Design review of the part shown in the three views and the two pictorial views. Dimensions are in mm from the part's minimum x, y and z. Give positions to 0.01 mm unless a question says otherwise; leave off trailing zeros. Loops run counter-clockwise (first coordinate to the right, second up) from the corner with the lowest first, then second, coordinate; pieces in that order, holes last. Notation, with made-up numbers: (35.25, -31.5) - (66.25, -31.5) arc R18 ccw to (66.25, -4.5) - close; hole circle Ø7 at (-34.5, -37). An arc over 180 degrees is marked (long way). Answer as a JSON object with one key per item and string values.
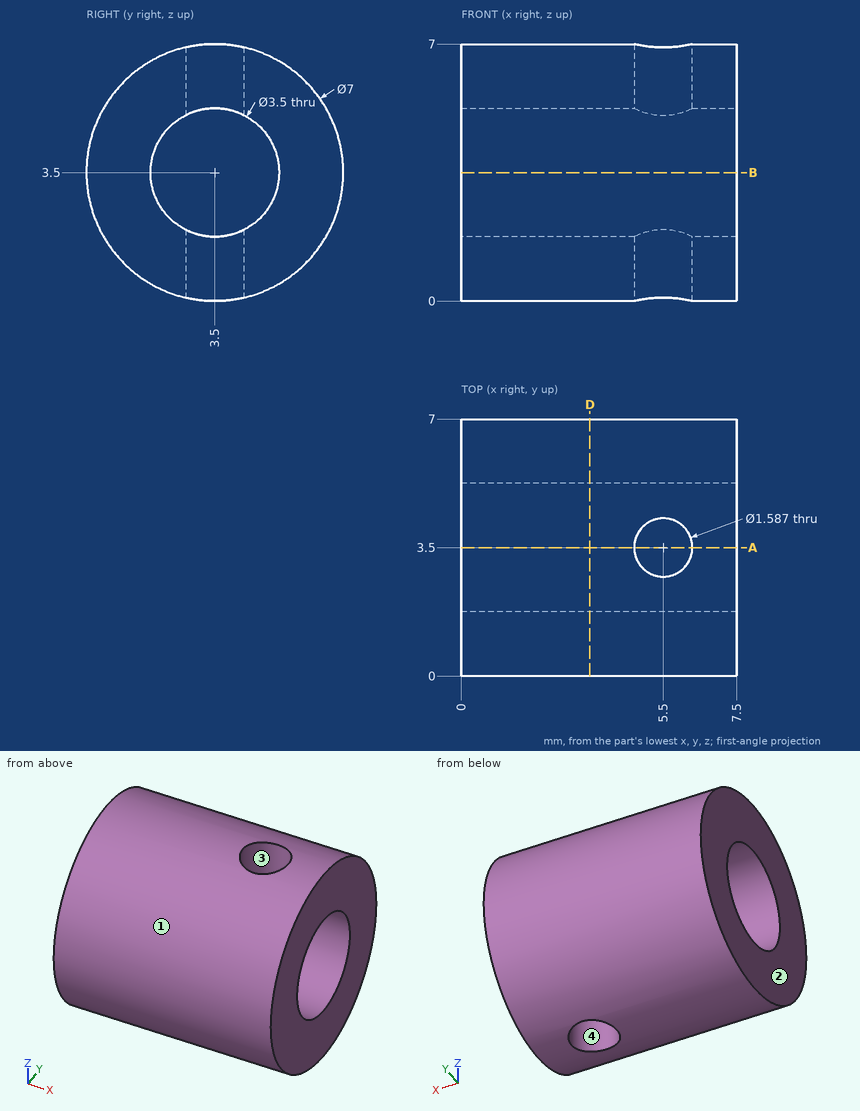
Q1. Consider section D-D, the plane x = 3.5. State the section outline as (y, z) points.
Results:
{"outline": "circle Ø7 at (3.5, 3.5); hole circle Ø3.5 at (3.5, 3.5)"}
Q2. Consider section B-B, the plane z = 3.5. State the section outline as (x, y) points.
Results:
{"outline": "(0, 0) - (7.5, 0) - (7.5, 1.75) - (0, 1.75) - close; (0, 5.25) - (7.5, 5.25) - (7.5, 7) - (0, 7) - close"}
Q3. To check wall thickness, follow probe 1 along Y at (x, z) = (4, 3.5); probe 2 along Z at (x, y) = (7.25, 4.5) (1 decimal); probe 3 along Z at (x, y) = (7.25, 5) (1 decimal). State the ranges of each line that lie inside material, in increasing order. Write a range as [from, to].
Results:
{"probe 1": "y = [0, 1.75], [5.25, 7]", "probe 2": "z = [0.1, 2.1], [4.9, 6.9]", "probe 3": "z = [0.3, 2.6], [4.4, 6.7]"}
Q4. The part is to be moulded in two halves that separate along Y. For the marked faces 1, 2, 3 and 4, say which applies: +Y half, -Y half, draft (parallel to the pull), parting line (faces both ways), or undercut.
Results:
{"face 1": "parting line", "face 2": "draft", "face 3": "undercut", "face 4": "undercut"}
Q5. Consider section A-A, the plane y = 3.5. State the section outline as (x, z) points.
Results:
{"outline": "(0, 0) - (4.71, 0) - (4.71, 1.75) - (0, 1.75) - close; (0, 5.25) - (4.71, 5.25) - (4.71, 7) - (0, 7) - close; (6.29, 0) - (7.5, 0) - (7.5, 1.75) - (6.29, 1.75) - close; (6.29, 5.25) - (7.5, 5.25) - (7.5, 7) - (6.29, 7) - close"}
